```python
from build123d import *

# Parameters (mm, degrees)
F1_DEPTH = 63.5
F2_DEPTH = 25.4
F3_DEPTH = 7.9375
F5_R     = 6.35


with BuildPart() as f1:
    # F0 (on Front) → F1 (new body, symmetric)
    with BuildSketch(Plane.XZ):
        Polygon((-41.275, -9.525), (41.275, -9.525), (41.275, 9.525), (22.225, 9.525), (-41.275, 9.525), align=None)
    extrude(amount=F1_DEPTH, both=True)

    # F0 (on Front) → F2 (join, symmetric)
    with BuildSketch(Plane.XZ):
        with BuildLine():
            Line((22.225, 9.525), (41.275, 9.525))
            Line((41.275, 9.525), (41.275, 27.0002))
            ThreePointArc((41.275, 27.0002), (45.92468, 38.22552), (57.15, 42.8752))
            Line((57.15, 42.8752), (60.325, 42.8752))
            Line((60.325, 42.8752), (60.325, 61.9252))
            Line((60.325, 61.9252), (57.15, 61.9252))
            add(Edge.make_bspline(
                [(56.025, 61.907076), (56.404449, 61.915352), (56.7795, 61.921393), (57.15, 61.9252)],
                knots=[110.209963, 110.209963, 110.209963, 110.209963, 111.504536, 111.504536, 111.504536, 111.504536], degree=3))
            ThreePointArc((56.025, 61.907076), (32.059701, 51.294901), (22.225, 27.0002))
            Line((22.225, 27.0002), (22.225, 9.525))
        make_face()
        Polygon((60.325, 61.9252), (60.325, 42.8752), (70.739483, 42.8752), (85.725, 42.8752), (85.725, 52.3875), (85.725, 61.9252), (70.739483, 61.9252), align=None)
    extrude(amount=F2_DEPTH, both=True)

    # F0 (on Front) → F3 (join, symmetric)
    with BuildSketch(Plane.XZ):
        with BuildLine():
            add(Edge.make_bspline(
                [(-41.275, 9.525), (-40.450122, 44.294677), (23.721684, 61.202513), (56.025, 61.907076)],
                knots=[0, 0, 0, 0, 110.209963, 110.209963, 110.209963, 110.209963], degree=3))
            Line((-41.275, 9.525), (22.225, 9.525))
            Line((22.225, 9.525), (22.225, 27.0002))
            ThreePointArc((22.225, 27.0002), (32.059701, 51.294901), (56.025, 61.907076))
        make_face()
    extrude(amount=F3_DEPTH, both=True)

    # F0 (on Front) → F4 (revolve)
    with BuildSketch(Plane.XZ):
        Polygon((85.725, 42.8752), (85.725, 38.1), (111.125, 38.1), (111.125, 66.675), (85.725, 66.675), (85.725, 61.9252), (85.725, 52.3875), align=None)
    revolve(axis=Axis((85.725, 0, 40.4876), (0, 0, -1)))

    # F5
    f5_edges = [f1.edges().sort_by_distance(p)[0] for p in [
        (-41.275, -63.5, 0),
        (41.275, -63.5, 0),
        (41.275, 63.5, 0),
        (-41.275, 63.5, 0),
    ]]
    fillet(f5_edges, radius=F5_R)


solid = f1.part
```
CAD build for the part. Positions are in the model's coordinates, mm. A direction names the side the tool comes from. Coordinates: 2 decimals unless noted, no trailing zeros. Order: outer loops, then holes, each group sorted by start corner. A loop starts at its lowest first (then second) coordinate and runs counter-clockwise, first axis right, second up. Notation, with made-up numbers: (29.25, -31.5) -> (63.25, -31.5) arc R19 cw to (63.25, -6.5) -> close; hole circle Ø2 at (86.25, 52.25). An arc over 180 degrees is marked (long way). Use one line per item in the form item = value. Start each with the question number.
1) Band-saw the part on A-A on z = 6.5. Give the cut face in (x, y) (3 decimals).
2) Band-saw the part on C-C on x = 91. Give the cut face in (y, z) (3 decimals).
3) Band-saw the part on B-B on y = 39. Give the cut face in (x, z) (3 decimals), then the cut area to 3 significant figures.
4) Drill centre lines: L1, parallel to X at y = -56.5, z = 1 (3 decimals); L2, parallel to Y at x = -24.5, z = 23.5; L3, parallel to Z at x = 2, y = 25.5 (3 decimals). Where is each one in solid material? Low to high. Write a range as [from, to].
5) Drop flat-ended pins along their axis: pin 1 (14 mm diameter, centred on y = 14.5, z = 16, fed in from -X) (3 decimals); pin 2 (15.5 mm diameter, centred on x = -12, z = 23, fed in from -Y); pin 3 (1.5 mm diameter, centred on y = 26.5, z = 51, fed in from +X); pin 4 (4 mm diameter, centred on x = 66, y = 16.5, fed in from -Z). Give the stop position or say it passes through.
6) Pull direction X, two halves, no side cores. Call faces 1 (the cylindrical face through (32.32, 16.55, 51.56)), 2 (the flat face through (60, 2, 42.875)), 3 (the cylindrical face through (39.464, 61.59, 0.133)): +X half, -X half, draft (parallel to the pull), parting line (faces both ways), or undercut.
7) Tool access for faces 4 (the flat face through (86, 0, 38.1)), 5 (the cylindrical face through (45.8, -0.4, 38.1)), 6 (the flat face through (-3, -7.938, 30)), 7 (the flat face through (46, -25.4, 42)), 8 (the flat face through (-3, 7.938, 30)): list every direction of +Z, -Z, +X, -X, +Y, -Y with a clear straight run to the whole face (end or side of a thin tool).
Entries:
q1.outline = (-41.275, -57.15) arc R6.35 ccw to (-34.925, -63.5) -> (34.925, -63.5) arc R6.35 ccw to (41.275, -57.15) -> (41.275, 57.15) arc R6.35 ccw to (34.925, 63.5) -> (-34.925, 63.5) arc R6.35 ccw to (-41.275, 57.15) -> close
q2.outline = (-24.846, 38.1) -> (24.846, 38.1) -> (24.846, 66.675) -> (-24.846, 66.675) -> close
q3.outline = (-41.275, -9.525) -> (41.275, -9.525) -> (41.275, 9.525) -> (-41.275, 9.525) -> close
q3.area = 1,570 mm2
q4.L1 = [-41.275, 41.275]
q4.L2 = [-7.94, 7.94]
q4.L3 = [-9.525, 9.525]
q5.pin_1 = -41.275
q5.pin_2 = -7.94
q5.pin_3 = through
q5.pin_4 = 38.1
q6.face_1 = -X half
q6.face_2 = undercut
q6.face_3 = +X half
q7.face_4 = -Z, +X, +Y, -Y
q7.face_5 = -Z, +Y, -Y
q7.face_6 = +Z, -X, -Y
q7.face_7 = +Z, +X, -X, -Y
q7.face_8 = +Z, -X, +Y
